Design review of the part shown in the three views and the two pictorial views. Dimensions are in mm from the part's minimum x, y and z. A direction names the side the tool comes from. Round coordinates to 2 decimals unless told otherwise and drop trailing zeros. Loops run counter-clockwise (first coordinate to the right, second up) from the corner with the lowest first, then second, coordinate; pieces in that order, holes last. Notation, with made-up numbers: (6, -9.75) -> (48, -9.75) arc R17 ccw to (48, 11.25) -> close; hole circle Ø7 at (10.25, 12.5). An arc over 180 degrees is marked (long way). One line per question, with ' | ' between items. Start each with the question number.
1. Consider section B-B (z = 16.5). Write out the cut boundary in (x, y).
2. For pin 1 Ø5 at (x, z) = (80, 131.5) entering from -Y; pin 2 Ø12 at (y, z) = (157, 127) entering from -X (1 decimal); pin 3 Ø3 at (x, z) = (64.5, 76.5) entering from -Y, all flat-tipped, find the tip position at first contact; note any pin that passes through.
3. Wall thickness on line 1 along Y through (x, z) = (57, 3); line 2 along Z through (x, y) = (39.5, 141); line 3 along Y through (x, z) = (61, 28): over which ranges is each line inside the solid? List them lowest first.
4. Draft analysis for pull direction X (two halves, no side actions). For the marked faces 6, 7 and 8, state which applies: pulls with the +X half, pulls with the -X half, needs draft (parallel to the pull), parting line crosses it, or undercut.
5. For the marked faces 1, 2, 3, 4 and 5, list the 3-axis set-ups (+Z, -Z, +X, -X, +Y, -Y) from which the entire face can be reached by the end or side of a thin tool; tool diameter is ignored.
6. Consider section A-A (x = 57.5). Write out the cut boundary in (y, z).
7. Consider section C-C (y = 120). Write out the cut boundary in (x, z).
8. Consider section D-D (x = 108.5). Write out the cut boundary in (y, z) (1 decimal), and give its area (3 significant figures).
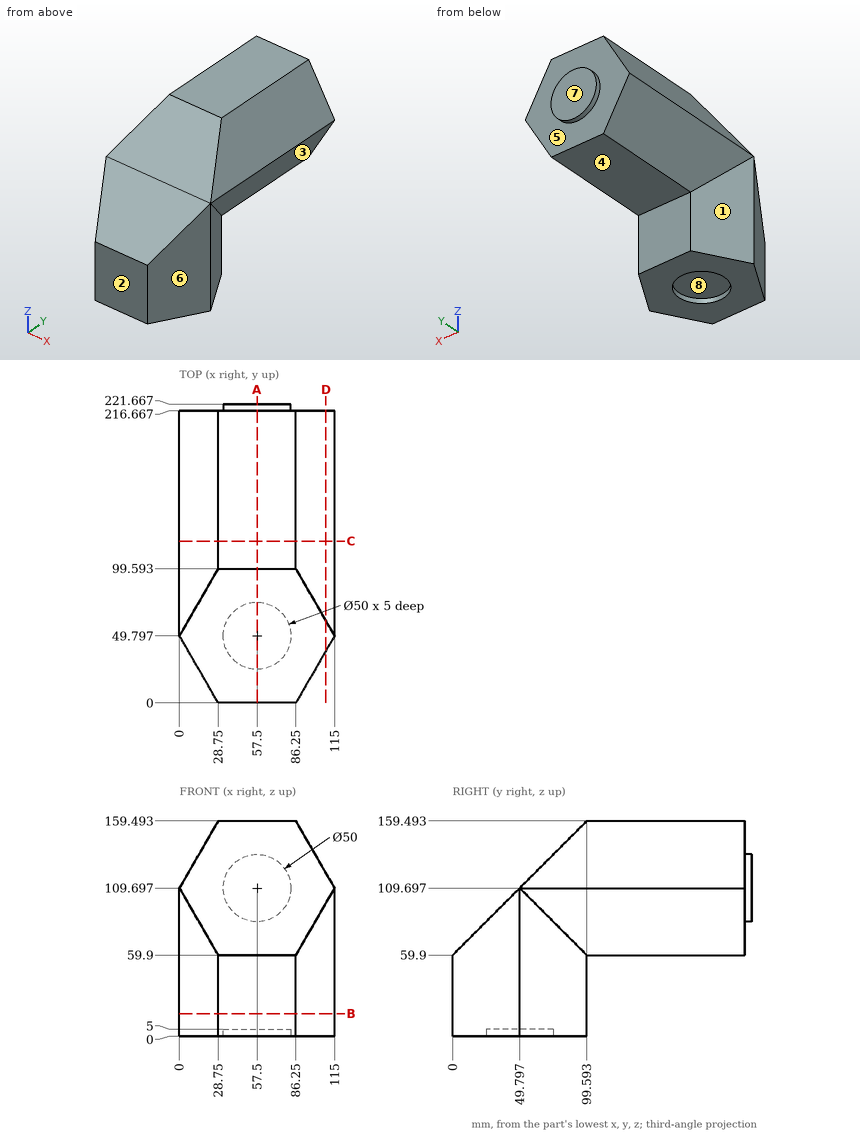
Answer block:
1) outline: (0, 49.8) -> (28.75, 0) -> (86.25, 0) -> (115, 49.8) -> (86.25, 99.59) -> (28.75, 99.59) -> close
2) pin 1: stops at y = 69.1 | pin 2: stops at x = 6.5 | pin 3: stops at y = 15.1
3) line 1: y = 0 to 24.8, 74.79 to 99.59 | line 2: z = 59.9 to 159.49 | line 3: y = 0 to 99.59
4) face 6: pulls with the +X half | face 7: needs draft | face 8: undercut
5) face 1: -Z, -X, +Y | face 2: +Z, -Z, +X, -X, -Y | face 3: -Z, +X, +Y | face 4: -Z, +X, -X, +Y | face 5: +Y
6) outline: (0, 0) -> (24.8, 0) -> (24.8, 5) -> (74.8, 5) -> (74.8, 0) -> (99.59, 0) -> (99.59, 59.9) -> (216.67, 59.9) -> (216.67, 84.7) -> (221.67, 84.7) -> (221.67, 134.7) -> (216.67, 134.7) -> (216.67, 159.49) -> (99.59, 159.49) -> (49.8, 109.7) -> (0, 59.9) -> close
7) outline: (0, 109.7) -> (28.75, 59.9) -> (86.25, 59.9) -> (115, 109.7) -> (86.25, 159.49) -> (28.75, 159.49) -> close
8) outline: (38.5, 0) -> (61.1, 0) -> (61.1, 98.4) -> (216.7, 98.4) -> (216.7, 121) -> (61.1, 121) -> (49.8, 109.7) -> (38.5, 98.4) -> close | area: 5,970 mm2
